Input: part model. Units: mm. Frame: model coordinates. Give positions to 0.01 mm unless a question says otherwise; leave off trailing zeros. Loops run counter-clockwise (first coordinate to the right, second up) from the corner with the lowest first, then second, coordinate; pieces in that order, holes last. Notation, with made-up numbers: (-29, 34.25) -> (-1, 34.25) arc R27 cw to (-1, 59.25) -> close; hole circle Ø8 at (-11, 66.5). An arc over 180 degrees is marked (long way). Answer as a JSON object with one key per item and string values. Group by question number.
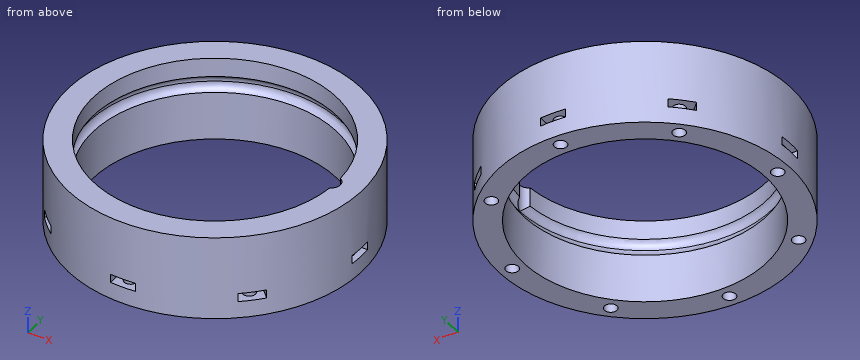
```python
from build123d import *

# Parameters (mm, degrees)
BOX060_W                    = 6
BOX060_H                    = 6
BOX060_DEPTH                = 2
BOX061_W                    = 6
BOX061_H                    = 6
BOX061_DEPTH                = 2
BOX061_PLACEMENT_ANGLE      = 135
BOX062_W                    = 6
BOX062_H                    = 6
BOX062_DEPTH                = 2
BOX063_W                    = 6
BOX063_H                    = 6
BOX063_DEPTH                = 2
BOX063_PLACEMENT_ANGLE      = 225
BOX064_W                    = 6
BOX064_H                    = 6
BOX064_DEPTH                = 2
BOX065_W                    = 6
BOX065_H                    = 6
BOX065_DEPTH                = 2
BOX065_PLACEMENT_ANGLE      = 45
BOX058_W                    = 6
BOX058_H                    = 6
BOX058_DEPTH                = 2
BOX059_W                    = 6
BOX059_H                    = 6
BOX059_DEPTH                = 2
BOX059_PLACEMENT_ANGLE      = 45
CYLINDER149_R               = 1.5
CYLINDER149_DEPTH           = 10
CYLINDER150_R               = 1.5
CYLINDER150_DEPTH           = 10
CYLINDER150_PLACEMENT_ANGLE = 135
CYLINDER151_R               = 1.5
CYLINDER151_DEPTH           = 10
CYLINDER152_R               = 1.5
CYLINDER152_DEPTH           = 10
CYLINDER152_PLACEMENT_ANGLE = 225
CYLINDER153_R               = 1.5
CYLINDER153_DEPTH           = 10
CYLINDER154_R               = 1.5
CYLINDER154_DEPTH           = 10
CYLINDER154_PLACEMENT_ANGLE = 45
CYLINDER147_R               = 1.5
CYLINDER147_DEPTH           = 10
CYLINDER148_R               = 1.5
CYLINDER148_DEPTH           = 10
CYLINDER148_PLACEMENT_ANGLE = 45
CYLINDER146_R               = 2.2
CYLINDER146_DEPTH           = 10
TORUS002_R                  = 2.2
TUBE009_R                   = 35
TUBE009_R_2                 = 29
TUBE009_DEPTH               = 20


with BuildPart() as krychle060:
    # Box060 → Box060 (new body)
    with BuildSketch(Plane(origin=(-29, -3, 14), x_dir=(0, 1, 0), z_dir=(0, 0, 1))):
        with Locations((3, 3)):
            Rectangle(BOX060_W, BOX060_H)
    extrude(amount=BOX060_DEPTH)


with BuildPart() as krychle061:
    # Box061 → Box061 (new body)
    with BuildSketch(Plane.XY):
        with Locations((3, 3)):
            Rectangle(BOX061_W, BOX061_H)
    extrude(amount=BOX061_DEPTH)


with BuildPart() as krychle061_1:
    # Box061 placement: moved
    add(krychle061.part.moved(Location((-18.384776, -22.627417, 14))).rotate(Axis((-18.384776, -22.627417, 14), (0, 0, 1)), BOX061_PLACEMENT_ANGLE))


with BuildPart() as krychle062:
    # Box062 → Box062 (new body)
    with BuildSketch(Plane(origin=(3, -29, 14), x_dir=(-1, 0, 0), z_dir=(0, 0, 1))):
        with Locations((3, 3)):
            Rectangle(BOX062_W, BOX062_H)
    extrude(amount=BOX062_DEPTH)


with BuildPart() as krychle063:
    # Box063 → Box063 (new body)
    with BuildSketch(Plane.XY):
        with Locations((3, 3)):
            Rectangle(BOX063_W, BOX063_H)
    extrude(amount=BOX063_DEPTH)


with BuildPart() as krychle063_1:
    # Box063 placement: moved
    add(krychle063.part.moved(Location((22.627417, -18.384776, 14))).rotate(Axis((22.627417, -18.384776, 14), (0, 0, 1)), BOX063_PLACEMENT_ANGLE))


with BuildPart() as krychle064:
    # Box064 → Box064 (new body)
    with BuildSketch(Plane(origin=(29, 3, 14), x_dir=(0, -1, 0), z_dir=(0, 0, 1))):
        with Locations((3, 3)):
            Rectangle(BOX064_W, BOX064_H)
    extrude(amount=BOX064_DEPTH)


with BuildPart() as krychle065:
    # Box065 → Box065 (new body)
    with BuildSketch(Plane.XY):
        with Locations((3, 3)):
            Rectangle(BOX065_W, BOX065_H)
    extrude(amount=BOX065_DEPTH)


with BuildPart() as krychle065_1:
    # Box065 placement: moved
    add(krychle065.part.moved(Location((18.384776, 22.627417, 14))).rotate(Axis((18.384776, 22.627417, 14), (0, 0, -1)), BOX065_PLACEMENT_ANGLE))


with BuildPart() as krychle058:
    # Box058 → Box058 (new body)
    with BuildSketch(Plane(origin=(-3, 29, 14), x_dir=(1, 0, 0), z_dir=(0, 0, 1))):
        with Locations((3, 3)):
            Rectangle(BOX058_W, BOX058_H)
    extrude(amount=BOX058_DEPTH)


with BuildPart() as compound048:
    # Box059 → Box059 (new body)
    with BuildSketch(Plane.XY):
        with Locations((3, 3)):
            Rectangle(BOX059_W, BOX059_H)
    extrude(amount=BOX059_DEPTH)


with BuildPart() as compound048_1:
    # Box059 placement: moved
    add(compound048.part.moved(Location((-22.627417, 18.384776, 14))).rotate(Axis((-22.627417, 18.384776, 14), (0, 0, 1)), BOX059_PLACEMENT_ANGLE))

    # Compound048: union Krychle060, Krychle061, Krychle062, Krychle063, Krychle064, Krychle065, Krychle058
    add(krychle060.part)
    add(krychle061_1.part)
    add(krychle062.part)
    add(krychle063_1.part)
    add(krychle064.part)
    add(krychle065_1.part)
    add(krychle058.part)


with BuildPart() as obj1:
    # Cylinder149 → Cylinder149 (new body)
    with BuildSketch(Plane(origin=(-32, 0, 10), x_dir=(0, 1, 0), z_dir=(0, 0, 1))):
        Circle(CYLINDER149_R)
    extrude(amount=CYLINDER149_DEPTH)


with BuildPart() as obj2:
    # Cylinder150 → Cylinder150 (new body)
    with BuildSketch(Plane.XY):
        Circle(CYLINDER150_R)
    extrude(amount=CYLINDER150_DEPTH)


with BuildPart() as obj2_1:
    # Cylinder150 placement: moved
    add(obj2.part.moved(Location((-22.627417, -22.627417, 10))).rotate(Axis((-22.627417, -22.627417, 10), (0, 0, 1)), CYLINDER150_PLACEMENT_ANGLE))


with BuildPart() as obj3:
    # Cylinder151 → Cylinder151 (new body)
    with BuildSketch(Plane(origin=(0, -32, 10), x_dir=(-1, 0, 0), z_dir=(0, 0, 1))):
        Circle(CYLINDER151_R)
    extrude(amount=CYLINDER151_DEPTH)


with BuildPart() as obj4:
    # Cylinder152 → Cylinder152 (new body)
    with BuildSketch(Plane.XY):
        Circle(CYLINDER152_R)
    extrude(amount=CYLINDER152_DEPTH)


with BuildPart() as obj4_1:
    # Cylinder152 placement: moved
    add(obj4.part.moved(Location((22.627417, -22.627417, 10))).rotate(Axis((22.627417, -22.627417, 10), (0, 0, 1)), CYLINDER152_PLACEMENT_ANGLE))


with BuildPart() as obj5:
    # Cylinder153 → Cylinder153 (new body)
    with BuildSketch(Plane(origin=(32, 0, 10), x_dir=(0, -1, 0), z_dir=(0, 0, 1))):
        Circle(CYLINDER153_R)
    extrude(amount=CYLINDER153_DEPTH)


with BuildPart() as obj6:
    # Cylinder154 → Cylinder154 (new body)
    with BuildSketch(Plane.XY):
        Circle(CYLINDER154_R)
    extrude(amount=CYLINDER154_DEPTH)


with BuildPart() as obj6_1:
    # Cylinder154 placement: moved
    add(obj6.part.moved(Location((22.627417, 22.627417, 10))).rotate(Axis((22.627417, 22.627417, 10), (0, 0, -1)), CYLINDER154_PLACEMENT_ANGLE))


with BuildPart() as obj7:
    # Cylinder147 → Cylinder147 (new body)
    with BuildSketch(Plane(origin=(0, 32, 10), x_dir=(1, 0, 0), z_dir=(0, 0, 1))):
        Circle(CYLINDER147_R)
    extrude(amount=CYLINDER147_DEPTH)


with BuildPart() as compound047:
    # Cylinder148 → Cylinder148 (new body)
    with BuildSketch(Plane.XY):
        Circle(CYLINDER148_R)
    extrude(amount=CYLINDER148_DEPTH)


with BuildPart() as compound047_1:
    # Cylinder148 placement: moved
    add(compound047.part.moved(Location((-22.627417, 22.627417, 10))).rotate(Axis((-22.627417, 22.627417, 10), (0, 0, 1)), CYLINDER148_PLACEMENT_ANGLE))

    # Compound047: union obj1, obj2, obj3, obj4, obj5, obj6, obj7
    add(obj1.part)
    add(obj2_1.part)
    add(obj3.part)
    add(obj4_1.part)
    add(obj5.part)
    add(obj6_1.part)
    add(obj7.part)


with BuildPart() as obj8:
    # Cylinder146 → Cylinder146 (new body)
    with BuildSketch(Plane(origin=(28, 0, 23.5), x_dir=(1, 0, 0), z_dir=(0, 0, 1))):
        Circle(CYLINDER146_R)
    extrude(amount=CYLINDER146_DEPTH)


with BuildPart() as obj9:
    # Torus002 → Torus002 (revolve)
    with BuildSketch(Plane(origin=(0, 0, 23.5), x_dir=(1, 0, 0), z_dir=(0, -1, 0))):
        with Locations((28, 0)):
            Circle(TORUS002_R)
    revolve(axis=Axis((0, 0, 23.5), (0, 0, 1)))


with BuildPart() as obj10:
    # Tube009 → Tube009 (new body)
    with BuildSketch(Plane.XY.offset(10)):
        Circle(TUBE009_R)
        Circle(TUBE009_R_2, mode=Mode.SUBTRACT)
    extrude(amount=TUBE009_DEPTH)

    # Cut052: cut obj9
    add(obj9.part, mode=Mode.SUBTRACT)

    # Cut053: cut obj8
    add(obj8.part, mode=Mode.SUBTRACT)

    # Cut054: cut Compound047
    add(compound047_1.part, mode=Mode.SUBTRACT)

    # Cut055: cut Compound048
    add(compound048_1.part, mode=Mode.SUBTRACT)


solid = obj10.part
```
Q1. Section A-A on y = -32. Return the cut outline in (x, z), then the cut area to 3 significant figures.
Q2. Ray query, probe 1 along X at (y, z) = (0, 18.1); probe 2 along X at (y, z) = (23, 18.75). Return the intervals inside material, ascending.
Q3. Pin query (flat end, axial travel): pin 1 Ø12 at (y, z) = (13.5, 13) entering from +X; pin 2 Ø2 at (y, z) = (5.5, 23.5) entering from +X; pin 3 Ø0.9 at (x, y) = (23, 23) entering from -Z; pin 4 Ø6 at (y, z) = (2, 19) entering from -X. Return the tip coordinate at first contact, or that it passes through.
Numbers:
{
 "1": {"outline": "(-14.18, 10) -> (-1.5, 10) -> (-1.5, 14) -> (-3, 14) -> (-3, 16) -> (-1.5, 16) -> (-1.5, 20) -> (1.5, 20) -> (1.5, 16) -> (3, 16) -> (3, 14) -> (1.5, 14) -> (1.5, 10) -> (14.18, 10) -> (14.18, 30) -> (-14.18, 30) -> close", "area": "531 mm²"},
 "2": {"probe 1": "x = -35 to -33.5, -30.5 to -29, 29 to 30.5, 33.5 to 35", "probe 2": "x = -26.38 to -24.08, -21.17 to -17.66, 17.66 to 21.17, 24.08 to 26.38"},
 "3": {"pin 1": "stops at x = 34.19", "pin 2": "stops at x = 34.71", "pin 3": "stops at z = 20", "pin 4": "stops at x = -35"}
}
